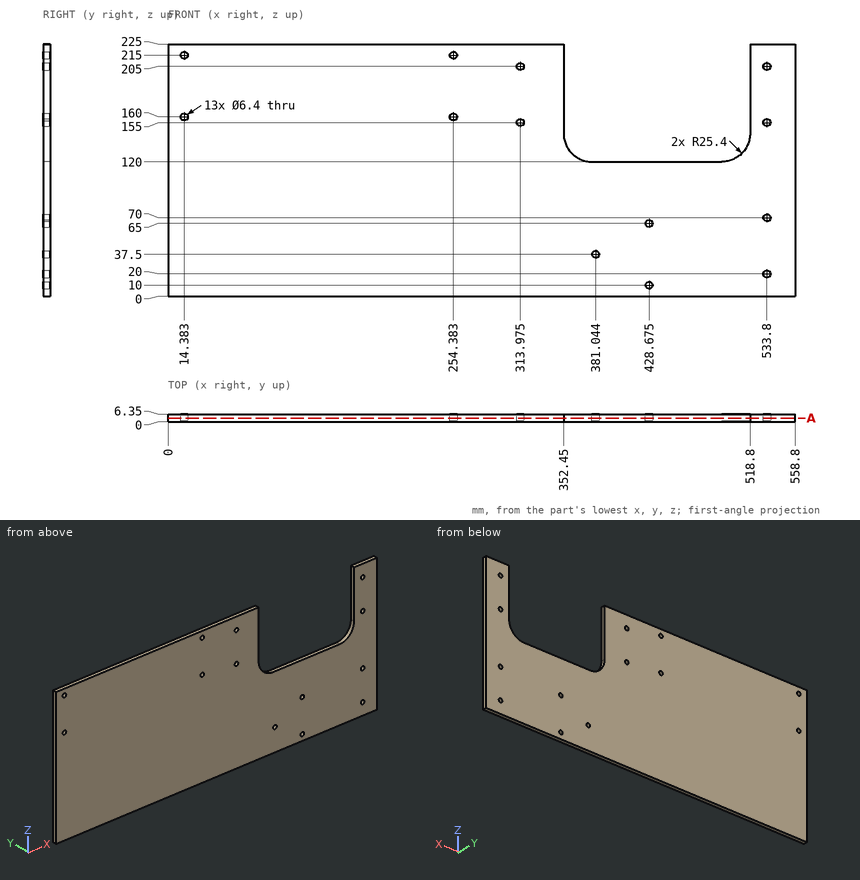
For this review, use the dimensioned drawing (mm, ordinates from the lowest corner) and the shaded views. Give positions to 0.01 mm unless a question says otherwise; leave off trailing zeros.
1) Insertion check: pin 1 (4 mm diameter, centred on x = 254.38, z = 160, fed in from -Y). The pin has a flat end and moves straight along its axis. Give the tip position at first contact, or say it passes through.
2) Take a section at A-A (y = 3). State how many separate pieces and enclosed holes the cut face has, then the cut area to 3 significant figures.
3) Wall thickness on line 1 (Z direction, x = 256.5, y = 2); line 2 (Z direction, x = 533.8, y = 2.5); line 3 (Z direction, x = 482, y = 6): over which ranges is each line inside the solid? List them lowest first.
Derived:
1. pin 1: passes through
2. separate pieces: 1
2. enclosed holes: 13
2. area: 108,000 mm2
3. line 1: z = 0 to 157.6, 162.4 to 212.6, 217.4 to 225
3. line 2: z = 0 to 16.8, 23.2 to 66.8, 73.2 to 151.8, 158.2 to 201.8, 208.2 to 225
3. line 3: z = 0 to 120
